Design review of the part built by this model. Coordinates are the model's own, in mm. Round coordinates to 2 decimals unless told otherwise and drop trailing zeros. Order: outer loops, then holes, each group sorted by start corner. A loop starts at its lowest first (then second) coordinate and runs counter-clockwise, first axis right, second up.
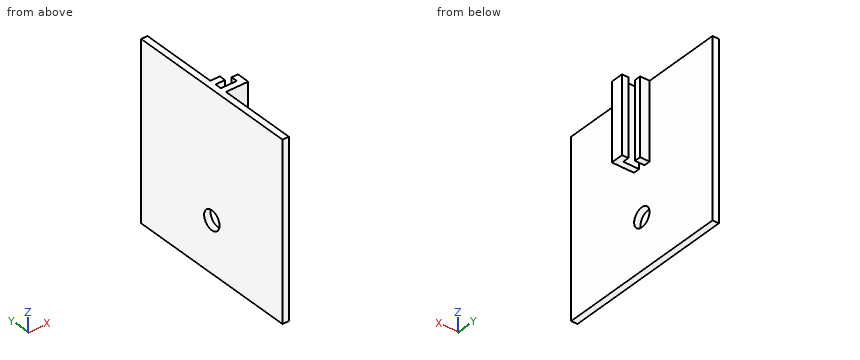
from build123d import *

# Parameters (mm, degrees)
SKETCH011_W     = 55.2
SKETCH011_H     = 55.2
SKETCH011_R     = 3
PAD007_DEPTH    = 2
SKETCH012_W     = 2
SKETCH012_H     = 24.2
PAD008_DEPTH    = 3
PAD008_FACE17_W = 2
PAD008_FACE17_H = 24.2
PAD010_DEPTH    = 4
SKETCH013_W     = 24.2
SKETCH013_H     = 2
PAD011_DEPTH    = 2


with BuildPart() as part:
    # Sketch011 (on DatumPlane) → Pad007 (new body)
    with BuildSketch(Plane(origin=(-57, 0, 0), x_dir=(0, 1, 0), z_dir=(-1, 0, 0))):
        with Locations((-89.497575, -0.4616)):
            Rectangle(SKETCH011_W, SKETCH011_H)
        with Locations((-89.497575, 11.1384)):
            Circle(SKETCH011_R, mode=Mode.SUBTRACT)
    extrude(amount=-PAD007_DEPTH)

    # Sketch012 (on Face7 of Pad007) → Pad008 (join)
    with BuildSketch(Plane.YZ.offset(-55)):
        with Locations((-87.447575, 15.9616)):
            Rectangle(SKETCH012_W, SKETCH012_H)
        with Locations((-91.547575, 15.9616)):
            Rectangle(SKETCH012_W, SKETCH012_H)
    extrude(amount=PAD008_DEPTH)

    # Pad008 Face17 → Pad010 (add)
    with BuildSketch(Plane(origin=(-52, -91.547575, 15.9616), x_dir=(0, -1, 0), z_dir=(1, 0, 0))):
        Rectangle(PAD008_FACE17_W, PAD008_FACE17_H)
    extrude(amount=PAD010_DEPTH)

    # Sketch013 (on Face20 of Pad010) → Pad011 (join)
    with BuildSketch(Plane(origin=(-57, -90.547575, 0), x_dir=(0, 0, -1), z_dir=(0, 1, 0))):
        with Locations((-15.9616, -8)):
            Rectangle(SKETCH013_W, SKETCH013_H)
    extrude(amount=PAD011_DEPTH)


solid = part.part
1) Take a section at B-B on z = 5. Give the boundary of the cut face in (x, y), plus the area to 3 significant figures.
Results:
outline: (-57, -117.1) - (-55, -117.1) - (-55, -92.55) - (-48, -92.55) - (-48, -88.55) - (-50, -88.55) - (-50, -90.55) - (-55, -90.55) - (-55, -88.45) - (-52, -88.45) - (-52, -86.45) - (-55, -86.45) - (-55, -61.9) - (-57, -61.9) - close
area: 134 mm2
2) Take a section at A-A on z = -13.5. Give the boundary of the cut face in (x, y).
Results:
outline: (-57, -117.1) - (-55, -117.1) - (-55, -91.35) - (-57, -91.35) - close; (-57, -87.65) - (-55, -87.65) - (-55, -61.9) - (-57, -61.9) - close
3) Take a section at D-D on x = -50.75. Give the boundary of the cut face in (y, z), plus the area to 3 significant figures.
Results:
outline: (-92.55, 3.86) - (-90.55, 3.86) - (-90.55, 28.06) - (-92.55, 28.06) - close
area: 48.4 mm2
4) Take a section at C-C on y = -112. Give the boundary of the cut face in (x, z).
Results:
outline: (-57, -27.14) - (-55, -27.14) - (-55, 28.06) - (-57, 28.06) - close
5) To check wall thickness, follow line 1 along Y through (x, z) = (-54.75, 14); line 2 along Y through (x, z) = (-50.75, 22); line 3 along Z through (x, y) = (-51.5, -91). State the ranges of each line that lie inside material, in increasing order.
Results:
line 1: y = -92.55 to -90.55, -88.45 to -86.45
line 2: y = -92.55 to -90.55
line 3: z = 3.86 to 28.06
6) Clearance check with flat-ended pins moving along their axes: P1, Ø2, axis at y = -99.5, z = -21, coming from the +X side; P2, Ø0.9, axis at x = -54, z = 10.5, coming from the -Y side; P3, Ø1.2, axis at x = -52.5, y = -90.5, coming from the -Z side. State where each tip first meets the part, or that it passes through.
Results:
P1: stops at x = -55
P2: stops at y = -92.55
P3: stops at z = 3.86
